For this review, take the finished solid that the model builds, in its own axes (mm). A direction names the side the tool comes from. Coordinates: 2 decimals unless noted, no trailing zeros. Write each loop counter-clockwise with the first axis right and the second up, starting at its lowest first coordinate (ties: lowest second). Pieces come first, ordered by that corner, then holes. Notation, with made-up numbers: M -21,-15 L 15,-15 A30 ccw 15,21 Z; hole C 66.5,31 d11. An arc over 180 degrees is marked long. Return JSON: item names as keys, results as strings.
```python
from build123d import *

# Parameters (mm, degrees)
BOSS_EXTRUDE1_DEPTH = 200
SKETCH2_R           = 3.75
CUT_EXTRUDE1_DEPTH  = 10
CUT_EXTRUDE2_DEPTH  = 10


with BuildPart() as part:
    # Sketch1 → Boss-Extrude1 (new body)
    with BuildSketch(Plane(origin=(0, 0, 0), x_dir=(1, 0, 0), z_dir=(0, 1, 0))):
        Polygon((10, 0), (10, 50), (10, 75), (0, 75), (0, 50), (0, 0), (0, -25), (10, -25), align=None)
    extrude(amount=BOSS_EXTRUDE1_DEPTH)

    # Sketch2 → Cut-Extrude1 (cut)
    with BuildSketch(Plane(origin=(10, 0, 0), x_dir=(0, 0, -1), z_dir=(1, 0, 0))):
        with Locations((25, 188.775303779)):
            Circle(SKETCH2_R)
        with Locations((25, 146.899681817)):
            Circle(SKETCH2_R)
    extrude(amount=-CUT_EXTRUDE1_DEPTH, mode=Mode.SUBTRACT)

    # Sketch3 → Cut-Extrude2 (cut)
    with BuildSketch(Plane.ZY):
        Polygon((25, 200), (25, 5), (10, 5), (0, 11.937821542), (0, 200), align=None)
        Polygon((-75, 5), (-60, 5), (-50, 11.937821542), (-50, 200), (-75, 200), align=None)
    extrude(amount=-CUT_EXTRUDE2_DEPTH, mode=Mode.SUBTRACT)


solid = part.part
```
1. Wall thickness on L1, parallel to Y at x = 3.25, z = -25; L2, parallel to Y at x = 6.25, z = -25.5; L3, parallel to Z at x = 9.25, y = 118: over which ranges is each line inside the solid? List them lowest first. Write a range as from..to.
Checks:
{"L1": "0..143.15, 150.65..185.03, 192.53..200", "L2": "0..143.18, 150.62..185.06, 192.49..200", "L3": "-50..0"}
2. For faces 4 (the face through (5, 105, -50)), 5 (the face through (10, 99, -24)), 6 (the face through (5, 105, 0)), list the 3-axis set-ups (+Z, -Z, +X, -X, +Y, -Y) from which the entire face can be reached by the end or side of a thin tool; tool diameter is ignored.
Checks:
{"face 4": "-Z, +X, -X, +Y", "face 5": "+Z, -Z, +X, +Y, -Y", "face 6": "+Z, +X, -X, +Y"}
3. We need section B-B (x = 6). State the section outline as (y, z) points.
Checks:
{"outline": "M 0,-75 L 5,-75 L 5,-60 L 11.94,-50 L 200,-50 L 200,0 L 11.94,0 L 5,10 L 5,25 L 0,25 Z; hole C 146.9,-25 d7.5; hole C 188.78,-25 d7.5"}
4. We need section A-A (z = -25). State the section outline as (x, y) points.
Checks:
{"outline": "M 0,0 L 10,0 L 10,143.15 L 0,143.15 Z; M 0,150.65 L 10,150.65 L 10,185.03 L 0,185.03 Z; M 0,192.53 L 10,192.53 L 10,200 L 0,200 Z"}
5. Clearance check with flat-ended pins moving along their axes: pin 1 Ø5 at (x, y) = (5.5, 106) entering from -Z; pin 2 Ø3 at (x, z) = (7, -67) entering from +Y; pin 3 Ø5 at (x, y) = (3.5, 112) entering from +Z. State where each tip first meets the part, or that it passes through.
Checks:
{"pin 1": "z = -50", "pin 2": "y = 5", "pin 3": "z = 0"}
6. Draft analysis for pull direction Y (two halves, no side actions). For faces 1 (the face through (5, 2, 25)), 2 (the face through (5.07, 143.24, -24.19)), 3 (the face through (4.9, 8.4, 5.1)), state which applies: +Y half, -Y half, draft (parallel to the pull), parting line (faces both ways), or undercut.
Checks:
{"face 1": "draft", "face 2": "undercut", "face 3": "+Y half"}
7. We need section C-C (y = 135). State the section outline as (x, z) points.
Checks:
{"outline": "M 0,-50 L 10,-50 L 10,0 L 0,0 Z"}
